Part print with two shaded views. Sizes in mm from the minimum x, y, z corner. Round coordinates to 2 decimals unless told otherwise and drop trailing zeros. Loops run counter-clockwise (first coordinate to the right, second up) from the corner with the lowest first, then second, coordinate; pieces in that order, holes last. Notation, with made-up numbers: (27.5, -28.75) - (47.5, -28.75) arc R17 ccw to (47.5, -2.75) - close; hole circle Ø8 at (48, 5). An arc over 180 degrees is marked (long way). Write each question's results on one line, items separated by ' | '. Start each with the question number.
(1) Cut at C-C, the plane y = 2.75. List the corners of the cut face in (x, z), then the cut area to 3 significant figures.
(2) Flat gauge pins, fed straight in: P1, Ø2, axis at x = 5.5, z = 14.5, coming from the +Y side; P2, Ø2.5, axis at y = 8.5, z = 13, coming from the -X side; P3, Ø4.5, axis at x = 5, z = 6.5, coming from the +Y side. Where does each tip first touch, or does it go through?
(3) Cut at D-D, the plane x = 1. List the corners of the cut face in (y, z), then the cut area to 3 significant figures.
(4) Cut at A-A, the plane x = 5. List the corners of the cut face in (y, z).
(5) Cut at B-B, the plane z = 30. List the corners of the cut face in (x, y).
(6) Drill centre lines: L1, parallel to Y at x = 5.25, z = 13.5; L2, parallel to Y at x = 1, z = 30; L3, parallel to X at y = 3, z = 19.5. Where is each one in solid material? Low to high.
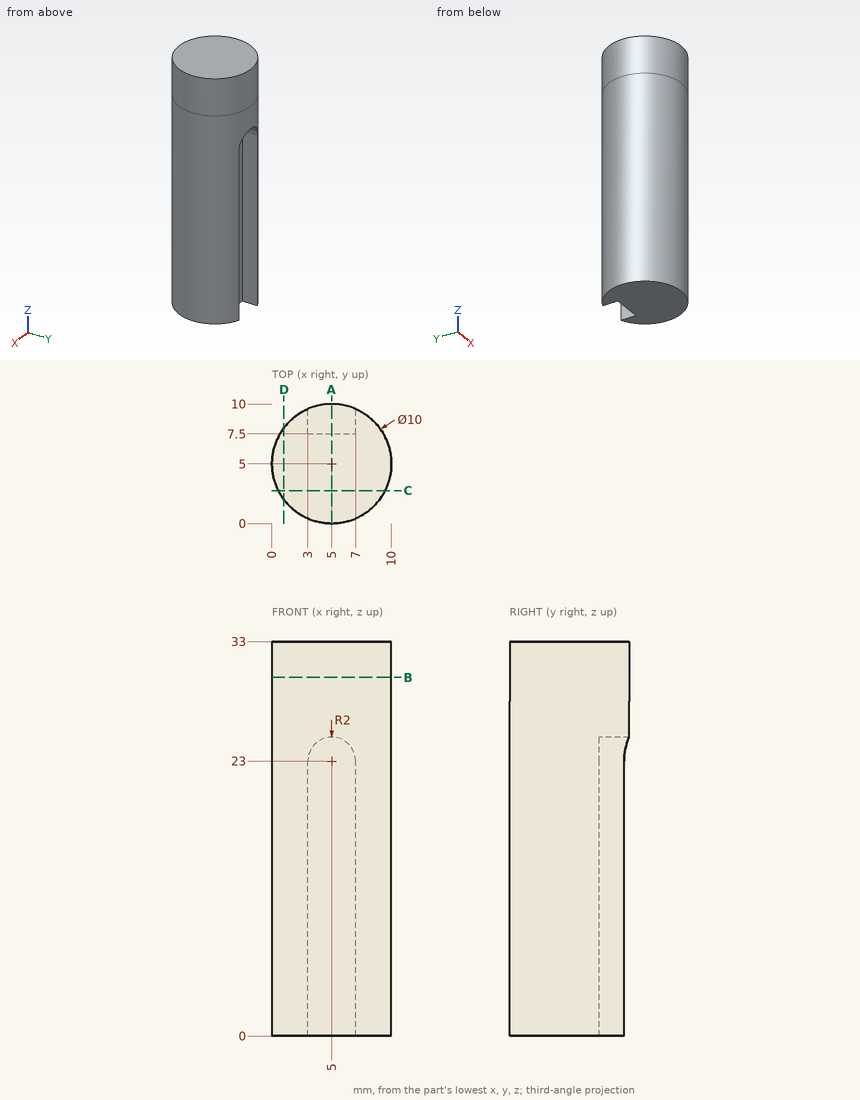
A:
1) outline: (0.53, 0) - (9.47, 0) - (9.47, 33) - (0.53, 33) - close | area: 295 mm2
2) P1: y = 7.5 | P2: x = 0.53 | P3: y = 9.58
3) outline: (2, 0) - (8, 0) - (8, 33) - (2, 33) - close | area: 198 mm2
4) outline: (0, 0) - (7.5, 0) - (7.5, 25) - (10, 25) - (10, 33) - (0, 33) - close
5) outline: circle Ø10 at (5, 5)
6) L1: 0.01 to 7.5 | L2: 2 to 8 | L3: 0.42 to 9.58
